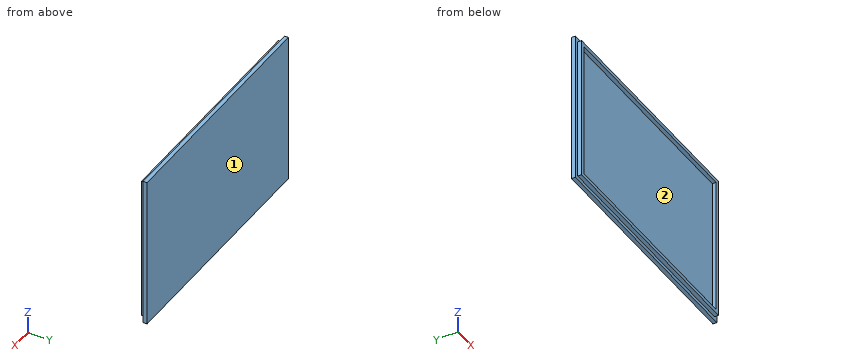
Autodesk Inventor part; units mm, degrees
ref_plane "Work Plane1" through (-93, 0, -56.8) normal (0, 0, 1) x (1, 0, 0)
ref_plane "YZ Plane" through (0, 0, 0) normal (1, 0, 0) x (0, 1, 0)
ref_plane "XZ Plane" through (0, 0, 0) normal (0, 1, 0) x (-1, 0, 0)
sketch "Sketch1" plane through (0, 0, 0) normal (0, 1, 0) x (-1, 0, 0)
  line L0 (90, -113.6) -> (-90, -113.6)
  line L1 (-90, -113.6) -> (-90, 0)
  line L2 (-90, 0) -> (90, 0)
  line L3 (90, 0) -> (90, -113.6)
  line L4 (-93, -116.6) -> (93, -116.6)
  line L5 (93, -116.6) -> (93, 3)
  line L6 (93, 3) -> (-93, 3)
  line L7 (-93, 3) -> (-93, -116.6)
  point P0 (0, 0)
  point P1 (0, 0)
  dimension "d0" = 180
  dimension "d1" = 113.6
  dimension "d2" = 3
extrude "Extrusion1" add sketch "Sketch1" along normal blind 3 contours L0 L1 L2 L3 | L7 L6 L5 L4
extrude "Extrusion2" add sketch "Sketch1" against normal blind 3 contours L0 L1 L2 L3
ref_plane "Work Plane1" through (-93, 0, -56.8) normal (0, 0, 1) x (1, 0, 0)
sketch "Sketch2" plane through (-93, 0, -56.8) normal (0, 0, 1) x (1, 0, 0)
  line L0 (0, 3) -> (186, 3)
  line L1 (159.34, 3) -> (146.166, 3)
  line L2 (146.166, 3) -> (142.9018, 10)
  line L3 (142.9018, 10) -> (162.6042, 10)
  line L4 (162.6042, 10) -> (159.34, 3)
  line L5 (119.506, 3) -> (106.332, 3)
  line L6 (106.332, 3) -> (103.0678, 10)
  line L7 (103.0678, 10) -> (122.7702, 10)
  line L8 (122.7702, 10) -> (119.506, 3)
  line L9 (93, 3) -> (93, -12.5812) construction
  line L10 (26.66, 3) -> (39.834, 3)
  line L11 (39.834, 3) -> (43.0982, 10)
  line L12 (43.0982, 10) -> (23.3958, 10)
  line L13 (23.3958, 10) -> (26.66, 3)
  line L14 (66.494, 3) -> (79.668, 3)
  line L15 (79.668, 3) -> (82.9322, 10)
  line L16 (82.9322, 10) -> (63.2298, 10)
  line L17 (63.2298, 10) -> (66.494, 3)
  point P0 (93, 0)
  point P1 (26.66, 3)
  point P2 (39.834, 3)
  point P3 (66.494, 3)
  point P4 (79.668, 3)
  dimension "d7" = 13.174
  dimension "d8" = 13.174
  dimension "d9" = 65
  dimension "d10" = 65
  dimension "d11" = 7
  dimension "d12" = 26.66
  dimension "d13" = 26.66
extrude "Extrusion3" [suppressed]
sketch "Sketch3" plane through (0, -3, 0) normal (0, -1, 0) x (1, 0, 0)
  line L0 (-87, -3) -> (87, -3)
  line L1 (87, -3) -> (87, -110.6)
  line L2 (87, -110.6) -> (-87, -110.6)
  line L3 (-87, -110.6) -> (-87, -3)
  line L4 (90, 0) -> (-90, 0)
  line L5 (-90, 0) -> (-90, -113.6)
  line L6 (-90, -113.6) -> (90, -113.6)
  line L7 (90, -113.6) -> (90, 0)
  point P0 (0, 0)
  dimension "d16" = 3
  dimension "d17" = 3
  dimension "d18" = 3
  dimension "d19" = 3
extrude "Extrusion4" cut sketch "Sketch3" against normal blind 3 contours L0 L1 L2 L3
properties part number "Lid"
Work out the finished part from the listing and answer in its coordinate system (mm). Face numbers are marked on the shaded views. Give positions to 0.01 mm unless a question says otherwise; leave off trailing zeros. Loops run counter-clockwise (first coordinate to the right, second up) from the corner with the lowest first, then second, coordinate; pieces in that order, holes last. Notation, with made-up numbers: (79, 29.25) - (102, 29.25) arc R12 cw to (102, 38.25) - close; hole circle Ø3 at (26, 42.25). An arc over 180 degrees is marked (long way). Answer in a Markdown table with one row per item. Add a question column.
Q1. The part is cut by section B-B (x = 20). Determine the outline of the cut face in (y, z).
Q2. Each of these flat-tipped pins is pushed along its axis until it touches: P1, Ø1.5, axis at x = 14, y = -1, coming from the -Z side; P2, Ø3, axis at x = -51.5, y = -2, coming from the +Z side; P3, Ø1, axis at x = -1.5, z = -69, coming from the -Y side. Where does it stop, or does it pass through?
Q3. Determine the mould class of the marked faces 1 and 2 for opening direction X: released by +X, released by -X, zero draft, split by the parting line, or undercut.
Q4. Consider line 1 along X through (y, z) = (-0.7, -7); line 2 along Z through (x, y) = (-33.5, -2.2); line 3 along Y through (x, z) = (-46, -60). Determine where each line is inside the solid, lowest interval first.
Q5. The part is cut by section A-A (z = -9). Determine the outline of the cut face in (x, y).
Solution:
| question | item | result |
|---|---|---|
| 1 | outline | (-3, -113.6) - (0, -113.6) - (0, -116.6) - (3, -116.6) - (3, 3) - (0, 3) - (0, 0) - (-3, 0) - (-3, -3) - (0, -3) - (0, -110.6) - (-3, -110.6) - close |
| 2 | P1 | stops at z = -113.6 |
| 2 | P2 | stops at z = 0 |
| 2 | P3 | stops at y = 0 |
| 3 | face 1 | zero draft |
| 3 | face 2 | undercut |
| 4 | line 1 | x = -90 to -87, 87 to 90 |
| 4 | line 2 | z = -113.6 to -110.6, -3 to 0 |
| 4 | line 3 | y = 0 to 3 |
| 5 | outline | (-93, 0) - (-90, 0) - (-90, -3) - (-87, -3) - (-87, 0) - (87, 0) - (87, -3) - (90, -3) - (90, 0) - (93, 0) - (93, 3) - (-93, 3) - close |
